```python
from build123d import *

# Parameters (mm, degrees)
SKETCH_1_W          = 31.99999989
SKETCH_1_H          = 11.5
SKETCH_1_R          = 2.2
EXTRUDE_1_DEPTH     = 29.5
SKETCH_2_R          = 2.5
CUT_EXTRUDE_1_DEPTH = 29.5
SKETCH_3_R          = 1.5
CUT_EXTRUDE_2_DEPTH = 29.5
CHAMFER_1_SIZE      = 1.5
SKETCH2_R           = 1.35
CUT_EXTRUDE1_DEPTH  = 10
EXTRUDE1_DEPTH      = 25


with BuildPart() as part:
    # 草图1 → 凸台-拉伸1 (new body)
    with BuildSketch(Plane.XY):
        with Locations((17.999999945, -43.99)):
            Rectangle(SKETCH_1_W, SKETCH_1_H)
        with Locations((8, -41.74)):
            Circle(SKETCH_1_R, mode=Mode.SUBTRACT)
        with Locations((27.99999989, -41.737899898)):
            Circle(SKETCH_1_R, mode=Mode.SUBTRACT)
    extrude(amount=EXTRUDE_1_DEPTH)

    # 草图2 → 切除-拉伸1 (cut)
    with BuildSketch(Plane.XZ.offset(49.74)):
        with Locations(Location((17.999999945, 14.75, 0), (0, 0, 270))):
            Circle(SKETCH_2_R)
    extrude(amount=-CUT_EXTRUDE_1_DEPTH, mode=Mode.SUBTRACT)

    # 草图3 → 切除-拉伸2 (cut)
    with BuildSketch(Plane.XZ.offset(49.74)):
        with Locations(Location((17.999999945, 8.75, 0), (0, 0, 270))):
            Circle(SKETCH_3_R)
        with Locations(Location((17.999999945, 20.75, 0), (0, 0, 270))):
            Circle(SKETCH_3_R)
    extrude(amount=-CUT_EXTRUDE_2_DEPTH, mode=Mode.SUBTRACT)

    # 倒角1
    chamfer_1_edges = [part.edges().sort_by_distance(p)[0] for p in [
        (17.999999945, -38.24, 10.25),
        (17.999999945, -38.24, 22.25),
    ]]
    chamfer(chamfer_1_edges, length=CHAMFER_1_SIZE)

    # Sketch2 → Cut-Extrude1 (cut)
    with BuildSketch(Plane(origin=(33.99999989, 0, 0), x_dir=(0, 0, -1), z_dir=(1, 0, 0))):
        with Locations((-19.5, -45.74)):
            Circle(SKETCH2_R)
        with Locations((-8, -45.74)):
            Circle(SKETCH2_R)
    cut_extrude1 = extrude(amount=-CUT_EXTRUDE1_DEPTH, mode=Mode.SUBTRACT)

    # Mirror1: Cut-Extrude1 across plane
    add(cut_extrude1.mirror(Plane.ZY.offset(-17.999999945)), mode=Mode.SUBTRACT)

    # Sketch3 → Extrude1 (cut)
    with BuildSketch(Plane(origin=(0, -38.24, 0), x_dir=(1, 0, 0), z_dir=(0, 1, 0))):
        with BuildLine():
            Line((11.2, 0), (13.653738644, -4.25))
            ThreePointArc((13.653738644, -4.25), (14.20277675, -4.799038106), (14.95277675, -5))
            Line((14.95277675, -5), (21.04722314, -5))
            ThreePointArc((21.04722314, -5), (21.79722314, -4.799038106), (22.346261246, -4.25))
            Line((22.346261246, -4.25), (24.79999989, 0))
            Line((24.79999989, 0), (11.2, 0))
        make_face()
        with BuildLine():
            Line((11.2, -29.5), (24.79999989, -29.5))
            Line((24.79999989, -29.5), (22.346261246, -25.25))
            ThreePointArc((22.346261246, -25.25), (21.79722314, -24.700961894), (21.04722314, -24.5))
            Line((21.04722314, -24.5), (14.95277675, -24.5))
            ThreePointArc((14.95277675, -24.5), (14.20277675, -24.700961894), (13.653738644, -25.25))
            Line((13.653738644, -25.25), (11.2, -29.5))
        make_face()
    extrude(amount=-EXTRUDE1_DEPTH, mode=Mode.SUBTRACT)


solid = part.part
```
Can you work these out from the model? Positions are in its coordinate system, mm. A direction names the side the tool comes from. Coordinates: 2 decimals unless noted, no trailing zeros. Loops run counter-clockwise (first coordinate to the right, second up) from the corner with the lowest first, then second, coordinate; pieces in that order, holes last. Notation, with made-up numbers: (39, 80) -> (53, 80) arc R16 ccw to (53, 93) -> close; hole circle Ø7 at (21.25, 87.5). An arc over 180 degrees is marked (long way). Answer as a JSON object with one key per item and string values.
1) Imagine slicing it at C-C (z = 8.75). Please give me the cut outline in (x, y).
Results:
{"outline": "(2, -49.74) -> (16.5, -49.74) -> (16.5, -39.74) -> (15, -38.24) -> (2, -38.24) -> (2, -44.62) -> (12, -44.62) -> (12, -46.86) -> (2, -46.86) -> close; (19.5, -49.74) -> (34, -49.74) -> (34, -46.86) -> (24, -46.86) -> (24, -44.62) -> (34, -44.62) -> (34, -38.24) -> (21, -38.24) -> (19.5, -39.74) -> close; hole circle Ø4.4 at (8, -41.74); hole circle Ø4.4 at (28, -41.74)"}
2) Thinking about a two-plate mould opening in Z: for faces 1 (the face through (14.212, -43.91, 24.695)), 2 (the face through (14.19, -43.91, 4.79)), 3 (the face through (29.07, -44.401, 8.176)), which applies, pulls with the +Z half, pulls with the -Z half, needs draft (parallel to the pull), parting line crosses it, or undercut?
Results:
{"face 1": "pulls with the +Z half", "face 2": "pulls with the -Z half", "face 3": "undercut"}
3) For faces 4 (the face through (24, -46, 20)), 5 (the face through (29.18, -39.88, 14.54)), 6 (the face through (23.59, -43.91, 27.405)), 7 (the face through (12, -46, 8)), 8 (the face through (21.788, -43.91, 4.805)), which set-ups out of +Z, -Z, +X, -X, +Y, -Y let a thin tool reach every point of the face, with its end or its side?
Results:
{"face 4": "+X", "face 5": "+Z, -Z", "face 6": "+Z, +Y, -Y", "face 7": "-X", "face 8": "-Z, +Y, -Y"}
4) Imagine slicing it at D-D (y = -45.25). Count the separate pieces of the cut face and the enclosed holes in it, then the cut area to 3 significant figures.
Results:
{"separate pieces": "1", "enclosed holes": "3", "area": "703 mm^2"}
5) If I drill on line 1 (Z direction, x = 18, y = -47.25); line 2 (Y direction, x = 8, z = 9); line 3 (X direction, y = -43.5, z = 4.25), over which ranges is the centre line in solid material (lowest first)?
Results:
{"line 1": "z = 5 to 7.25, 10.25 to 12.25, 17.25 to 19.25, 22.25 to 24.5", "line 2": "y = -49.74 to -46.65, -44.83 to -43.94, -39.54 to -38.24", "line 3": "x = 2 to 6.68, 9.32 to 13.65, 22.35 to 26.68, 29.32 to 34"}
6) Imagine slicing it at A-A (x = 8). Please give me the cut outline in (y, z).
Results:
{"outline": "(-49.74, 0) -> (-43.94, 0) -> (-43.94, 29.5) -> (-49.74, 29.5) -> close; (-39.54, 0) -> (-38.24, 0) -> (-38.24, 29.5) -> (-39.54, 29.5) -> close; hole circle Ø2.7 at (-45.74, 8); hole circle Ø2.7 at (-45.74, 19.5)"}
7) For P1, Ø1.6, axis at y = -45.74, z = 19.5, coming from the +X side; P2, Ø0.8, axis at y = -46, z = 19.5, coming from the -X side; P3, Ø3, axis at x = 18.5, y = -46, coming from the -Z side, each with a flat end and sliding along its axis, tell me the tip position at first contact or that it passes through.
Results:
{"P1": "stops at x = 24", "P2": "stops at x = 12", "P3": "stops at z = 5"}
8) Imagine slicing it at B-B (z = 14.75). Please give me the cut outline in (x, y).
Results:
{"outline": "(2, -49.74) -> (15.5, -49.74) -> (15.5, -38.24) -> (2, -38.24) -> close; (20.5, -49.74) -> (34, -49.74) -> (34, -38.24) -> (20.5, -38.24) -> close; hole circle Ø4.4 at (8, -41.74); hole circle Ø4.4 at (28, -41.74)"}
